Job drawing, mm, ordinate dimensions from the low corner. One solid piece. A direction names the side the tool comes from. Coordinates: 2 decimals unless noted, no trailing zeros. Write each loop counter-clockwise with the first axis right and the second up, starting at its lowest first coordinate (ties: lowest second). Pieces come first, ordered by that corner, then holes.
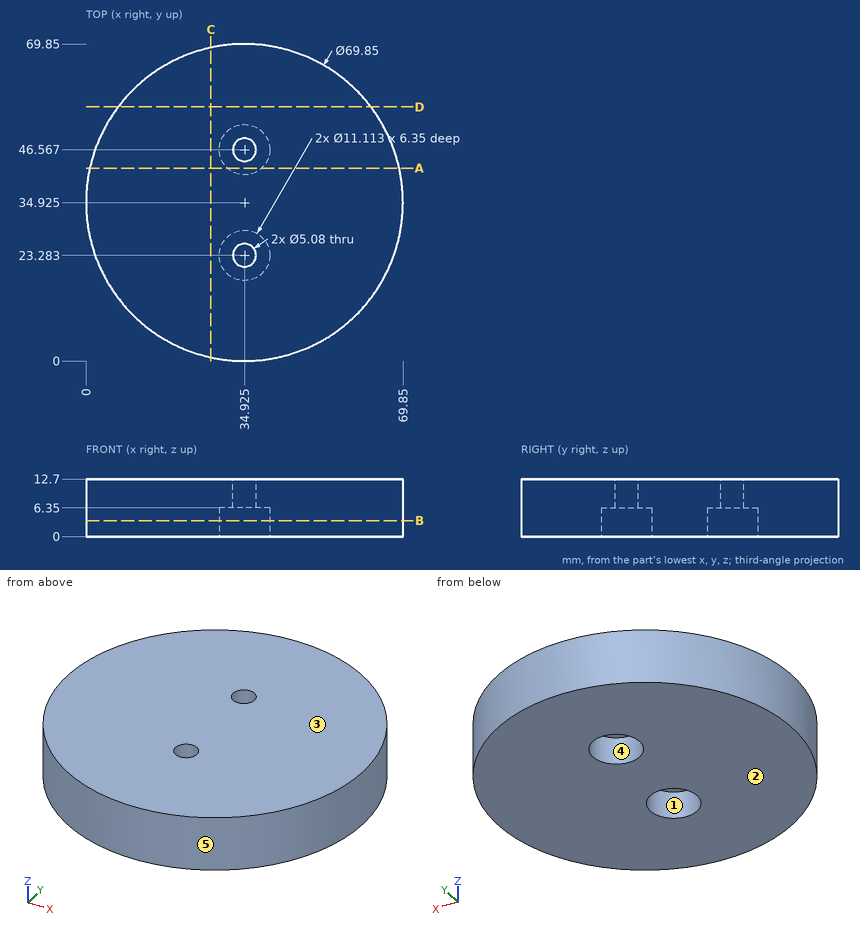
1. Saw through at B-B on z = 3.5. State how many separate pieces and enclosed holes the cut face has, plus the area to 3 significant figures.
Computed values:
separate pieces: 1
enclosed holes: 2
area: 3,640 mm2
2. 3-axis set-ups, long thin cutter, end or side, ignore diameter. For the marked faces 1 and 2: which of +Z, -Z, +X, -X, +Y, -Y reach the whole face in a straight line?
Computed values:
face 1: -Z
face 2: -Z, +X, -X, +Y, -Y
3. Saw through at D-D on y = 56. List the corners of the cut face in (x, z) (1 decimal).
Computed values:
outline: (7.1, 0) - (62.8, 0) - (62.8, 12.7) - (7.1, 12.7) - close
4. Saw through at A-A on y = 42.5. List the corners of the cut face in (x, z), plus the area to 3 significant figures.
Computed values:
outline: (0.83, 0) - (31.14, 0) - (31.14, 6.35) - (38.71, 6.35) - (38.71, 0) - (69.02, 0) - (69.02, 12.7) - (0.83, 12.7) - close
area: 818 mm2
5. Mould opens along Y. For the marked faces 3, 4 and 5 say: +Y half, -Y half, draft (parallel to the pull), parting line (faces both ways), or undercut.
Computed values:
face 3: draft
face 4: undercut
face 5: parting line
6. Saw through at C-C on x = 27.5. List the corners of the cut face in (y, z).
Computed values:
outline: (0.8, 0) - (69.05, 0) - (69.05, 12.7) - (0.8, 12.7) - close
7. Flat gauge pins, fed straight in: pin 1 (4 mm diameter, centred on y = 23.5, z = 1.5, fed in from -X) (1 decimal); pin 2 (3 mm diameter, centred on x = 48, z = 10, fed in from +Y); pin 3 (6 mm diameter, centred on y = 24.5, z = 5, fed in from -X). Where does each tip first touch, or does it go through?
Computed values:
pin 1: stops at x = 1.3
pin 2: stops at y = 67.88
pin 3: stops at x = 0.8
8. Probe line 1 along X through (y, z) = (34, 8.75); line 2 along X through (y, z) = (64, 11.25) (1 decimal); line 3 along Y through (x, z) = (5, 9) (1 decimal). List the from-to ranges inside material, lowest first.
Computed values:
line 1: x = 0.01 to 69.84
line 2: x = 15.6 to 54.3
line 3: y = 16.9 to 52.9
